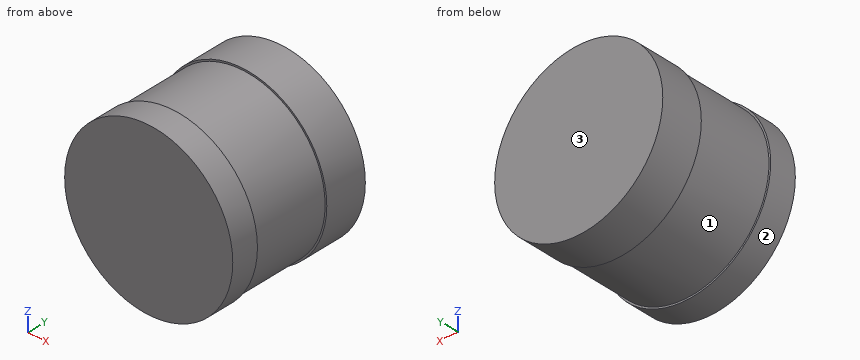
Autodesk Inventor part; units mm, degrees
ref_plane "작업 평면1" through (0, 61, 0) normal (0, 1, 0) x (1, 0, 0)
ref_plane "YZ Plane" through (0, 0, 0) normal (1, 0, 0) x (0, 1, 0)
ref_plane "XZ Plane" through (0, 0, 0) normal (0, 1, 0) x (-1, 0, 0)
sketch "스케치1" plane through (0, 0, 0) normal (0, 1, 0) x (-1, 0, 0)
  circle A0 centre (0, 0) radius 50
  dimension "d0" = 100
extrude "돌출1" add sketch "스케치1" along normal blind 86
ref_plane "작업 평면1" through (0, 61, 0) normal (0, 1, 0) x (1, 0, 0)
sketch "스케치2" plane through (0, 61, 0) normal (0, 1, 0) x (1, 0, 0)
  circle A0 centre (0, 0) radius 51.5789
  circle A1 centre (0, 0) radius 49
  dimension "d4" = 98
extrude "돌출2" cut sketch "스케치2" against normal blind 45
properties part number "lidar"
Model file for the job. Use its own axes, mm. Face numbers are marked on the shaded views. Give positions to 0.01 mm unless a question says otherwise; leave off trailing zeros. Order: outer loops, then holes, each group sorted by start corner. A loop starts at its lowest first (then second) coordinate and runs counter-clockwise, first axis right, second up. Notation, with made-up numbers: M -18,86 L 0,86 A32 ccw 0,120 Z; hole C 23.25,81.5 d3. An arc over 180 degrees is marked long. Put each result on its own line as item: value. Start each with the question number.
(1) Band-saw the part on A-A on z = -6. Give the cut face in (x, y), then the cut area to 3 significant figures.
(2) Band-saw the part on D-D on y = 65.5. Give the cut face in (x, z).
(3) Pin check, flat tips, straight feed: pin 1 Ø1 at (y, z) = (39, 4) entering from -X; pin 2 Ø2 at (y, z) = (64, -10) entering from +X; pin 3 Ø1 at (x, z) = (-8, 8) entering from -Y; pin 4 Ø1 at (y, z) = (75, -31.5) entering from -X. Stop position of each tip, or through.
(4) Pull direction Y, two halves, no side cores. Call the marked faces 1, 2 and 3: released by +Y, released by -Y, zero draft, split by the parting line, or undercut.
(5) Band-saw the part on C-C on y = 42. Give the cut face in (x, z), then the cut area to 3 significant figures.
(6) Drill centre lines: L1, parallel to X at y = 19, z = 26; L2, parallel to X at y = 31.5, z = 40. Where is each one in solid material? Low to high. Write a range as [from, to].
(7) Band-saw the part on B-B on x = 36.5. Give the cut face in (y, z).
Results below:
1. outline: M -49.64,0 L 49.64,0 L 49.64,16 L 48.63,16 L 48.63,61 L 49.64,61 L 49.64,86 L -49.64,86 L -49.64,61 L -48.63,61 L -48.63,16 L -49.64,16 Z
1. area: 8,450 mm2
2. outline: C 0,0 d100
3. pin 1: stops at x = -48.87
3. pin 2: stops at x = 49.18
3. pin 3: stops at y = 0
3. pin 4: stops at x = -39.23
4. face 1: undercut
4. face 2: zero draft
4. face 3: released by +Y
5. outline: C 0,0 d98
5. area: 7,540 mm2
6. L1: x = [-41.53, 41.53]
6. L2: x = [-28.3, 28.3]
7. outline: M 0,-34.17 L 16,-34.17 L 16,-32.69 L 61,-32.69 L 61,-34.17 L 86,-34.17 L 86,34.17 L 61,34.17 L 61,32.69 L 16,32.69 L 16,34.17 L 0,34.17 Z
